Build history of the part. All positions in model axes, mm. Face numbers are marked on the shaded views. A direction names the side the tool comes from. Round coordinates to 2 decimals unless told otherwise and drop trailing zeros. Order: outer loops, then holes, each group sorted by start corner. A loop starts at its lowest first (then second) coordinate and runs counter-clockwise, first axis right, second up. Notation, with made-up numbers: (-5, 78.5) -> (17, 78.5) arc R21 ccw to (17, 85.5) -> close; hole circle Ø6 at (22, 12). An arc over 180 degrees is marked (long way). Answer as a JSON object with one key per item and string values.
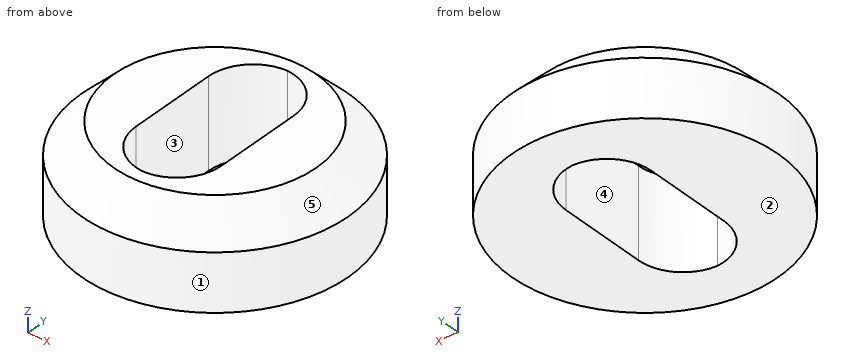
from build123d import *

# Parameters (mm, degrees)
F0_R        = 9.525
F0_W        = 6.096
F0_H        = 12.7
F1_DEPTH    = 6.35
F2_T1_DEPTH = 6.35
F3_SIZE     = 2.286


# Not quite as in the source:
# - a fillet or chamfer that OpenCascade refuses, or shapes differently, is made with other operations: its cross-section is extruded or revolved along the edge and cut away or added


with BuildPart() as f1:
    # F0 (on Top) → F1 (new body)
    with BuildSketch(Plane.XY):
        Circle(F0_R)
        Rectangle(F0_W, F0_H, mode=Mode.SUBTRACT)
    extrude(amount=F1_DEPTH)

    # F2: fillet of radius 3.1886932732 on 4 edges, made by hand

    # F2_s2 → F2_t1 (join)
    with BuildSketch(Plane.XY):
        with BuildLine():
            ThreePointArc((0.1406932732, 6.35), (-2.1140533634, 5.4160533634), (-3.048, 3.1613067268))
            Line((-3.048, 3.1613067268), (-3.048, 6.35))
            Line((-3.048, 6.35), (0.1406932732, 6.35))
        make_face()
        with BuildLine():
            ThreePointArc((-0.1406932732, 6.35), (2.1140533634, 5.4160533634), (3.048, 3.1613067268))
            Line((3.048, 3.1613067268), (3.048, 6.35))
            Line((3.048, 6.35), (-0.1406932732, 6.35))
        make_face()
        with BuildLine():
            ThreePointArc((0.1406932732, -6.35), (-2.1140533634, -5.4160533634), (-3.048, -3.1613067268))
            Line((-3.048, -3.1613067268), (-3.048, -6.35))
            Line((-3.048, -6.35), (0.1406932732, -6.35))
        make_face()
        with BuildLine():
            ThreePointArc((3.048, -3.1613067268), (2.1140533634, -5.4160533634), (-0.1406932732, -6.35))
            Line((-0.1406932732, -6.35), (3.048, -6.35))
            Line((3.048, -6.35), (3.048, -3.1613067268))
        make_face()
    extrude(amount=F2_T1_DEPTH)

    # F3
    f3_edges = [f1.edges().sort_by_distance(p)[0] for p in [
        (-9.525, 0, 6.35),
    ]]
    chamfer(f3_edges, length=F3_SIZE)


solid = f1.part
1) Flat gauge pins, fed straight in: pin 1 Ø3 at (y, z) = (1, 3) entering from +X (3 decimals); pin 2 Ø5 at (x, y) = (0.5, -1) entering from -Z. Where does each tip first touch, or does it go through?
Checked values:
{"pin 1": "stops at x = 9.525", "pin 2": "passes through"}
2) Cut at A-A, the plane y = 0. Give the cut face in (x, z) (3 decimals).
Checked values:
{"outline": "(-9.525, 0) -> (-3.048, 0) -> (-3.048, 6.35) -> (-7.239, 6.35) -> (-9.525, 4.064) -> close; (3.048, 0) -> (9.525, 0) -> (9.525, 4.064) -> (7.239, 6.35) -> (3.048, 6.35) -> close"}
3) Which spindle directions (+Z, -Z, +X, -X, +Y, -Y) get a long thin tool onto all of the face, cutting with end or side? Do the marked faces 4 and 5. Say none if no direction does.
Checked values:
{"face 4": "+Z, -Z", "face 5": "+Z"}
4) Probe L1, parallel to Y at x = -2.5, z = 0.75; L2, parallel to X at y = 1.75, z = 0.75; L3, parallel to X at y = -3.75, z = 4.75. List the from-to ranges inside material, lowest first. Write a range as from..to.
Checked values:
{"L1": "y = -9.19..-4.95, 4.95..9.19", "L2": "x = -9.36..-3.05, 3.05..9.36", "L3": "x = -8..-2.99, 2.99..8"}
5) Pull direction Y, two halves, no side cores. Call the marked faces 1, 2 and 3: pulls with the +Y half, pulls with the -Y half, needs draft (parallel to the pull), parting line crosses it, or undercut.
Checked values:
{"face 1": "parting line crosses it", "face 2": "needs draft", "face 3": "undercut"}
6) Cut at B-B, the plane z = 3.5. Give the cut face in (x, y) (3 decimals).
Checked values:
{"outline": "circle Ø19.05 at (0, 0); hole (-3.048, -3.161) arc R3.189 ccw to (0, -6.347) arc R3.189 ccw to (3.048, -3.161) -> (3.048, 3.161) arc R3.189 ccw to (0, 6.347) arc R3.189 ccw to (-3.048, 3.161) -> close"}
